Here's how the part is built. I have some questions about the finished solid (model axes, mm). A direction names the side the tool comes from. Coordinates: 2 decimals unless noted, no trailing zeros. Loops run counter-clockwise (first coordinate to the right, second up) from the corner with the lowest first, then second, coordinate; pieces in that order, holes last. Notation, with made-up numbers: (-10.5, -36.75) -> (34.5, -36.75) arc R27 ccw to (34.5, -1.75) -> close; hole circle Ø2 at (-15, 76.25). An arc over 180 degrees is marked (long way). Answer as a JSON object with one key per item and string values. Group by question number.
Q1. Thinking about a two-plate mould opening in X: for faces 1 (the flat face through (38.456, 19, 6)), 2 (the cylindrical face through (34.184, 23.722, 7.691)), 3 (the flat face through (19, 38.024, 6)), 4 (the flat face through (0, 19, 6)), which applies, released by +X, released by -X, zero draft, split by the parting line, or undercut?
Q2. On a 3-axis mill with a long thin cutter (end or side, diameter ignored), from which of +Z, -Z, +X, -X, +Y, -Y can I reach the whole of each face in a straight line? I mean faces 5 (the cylindrical face through (6.797, 18.465, 1.252)), 6 (the flat face through (15, 31, 2.54)). Say none if no direction works.
Q3. I need wall thicknesses on line 1 (X direction, y = 19, z = 7.5); line 2 (X direction, y = 19.5, z = 1); line 3 (Y direction, x = 31.5, z = 9.75). Which ranges of each line are inside material? Lowest first, please.
Q4. I want a section at A-A on y = 23.5. Write out the boundary of the cut face in (x, z), then the cut area to 3 significant figures.
Q5. I want a section at D-D on y = 33.5. Write out the boundary of the cut face in (x, z).
Q6. I want a section at C-C on z = 1. Write out the boundary of the cut face in (x, y).
Q7. I'm going to push a flat-ended pin straight in: pin 1 (15.5 mm diameter, centred on x = 17.5, y = 16, fed in from +Z). Where does the tip first touch, or does it pass through?
Q8. I want a section at B-B on x = 8.5. Write out the boundary of the cut face in (y, z), then the cut area to 4 significant figures.
```python
from build123d import *

# Parameters (mm, degrees)
F0_W     = 38.4559035301
F0_H     = 38.0239486694
F1_DEPTH = 12.7
F2_R     = 15.6804316887
F5_DEPTH = 10.16
F6_R     = 12.442666724
F7_DEPTH = 12.701


# Not quite as in the source:
# - the program builds the solid bodies; features that only make, move or delete a surface that nothing else refers to are left out


with BuildPart() as f1:
    # F0 (on Top) → F1 (new body)
    with BuildSketch(Plane.XY):
        with Locations((19.2279517651, 19.0119743347)):
            Rectangle(F0_W, F0_H)
    extrude(amount=F1_DEPTH)

    # F2 (on face) → F5 (cut)
    with BuildSketch(Plane.XY.offset(12.7)):
        with Locations((19.2279517651, 19.0119743347)):
            Circle(F2_R)
    extrude(amount=-F5_DEPTH, mode=Mode.SUBTRACT)

    # F6 (on face) → F7 (cut, through all)
    with BuildSketch(Plane(origin=(0, 0, 0), x_dir=(1, 0, 0), z_dir=(0, 0, -1))):
        with Locations((19.2279517651, -19.0119743347)):
            Circle(F6_R)
    extrude(amount=-F7_DEPTH, mode=Mode.SUBTRACT)


solid = f1.part
```
Result set:
{
 "1": {"face 1": "released by +X", "face 2": "undercut", "face 3": "zero draft", "face 4": "released by -X"},
 "2": {"face 5": "+Z, -Z", "face 6": "+Z"},
 "3": {"line 1": "x = 0 to 3.55, 34.91 to 38.46", "line 2": "x = 0 to 6.79, 31.66 to 38.46", "line 3": "y = 0 to 9.25, 28.77 to 38.02"},
 "4": {"outline": "(0, 0) -> (7.62, 0) -> (7.62, 2.54) -> (4.2, 2.54) -> (4.2, 12.7) -> (0, 12.7) -> close; (30.83, 0) -> (38.46, 0) -> (38.46, 12.7) -> (34.25, 12.7) -> (34.25, 2.54) -> (30.83, 2.54) -> close", "area": "124 mm²"},
 "5": {"outline": "(0, 0) -> (38.46, 0) -> (38.46, 12.7) -> (25.23, 12.7) -> (25.23, 2.54) -> (13.23, 2.54) -> (13.23, 12.7) -> (0, 12.7) -> close"},
 "6": {"outline": "(0, 0) -> (38.46, 0) -> (38.46, 38.02) -> (0, 38.02) -> close; hole circle Ø24.89 at (19.23, 19.01)"},
 "7": {"pin 1": "passes through"},
 "8": {"outline": "(0, 0) -> (12.71, 0) -> (12.71, 2.54) -> (7.58, 2.54) -> (7.58, 12.7) -> (0, 12.7) -> close; (25.32, 0) -> (38.02, 0) -> (38.02, 12.7) -> (30.45, 12.7) -> (30.45, 2.54) -> (25.32, 2.54) -> close", "area": "218.5 mm²"}
}
